```python
from build123d import *

# Parameters (mm, degrees)
SKETCH1_R                   = 60
SKETCH1_R_2                 = 37
BOSS_EXTRUDE1_DEPTH         = 4
F_3_16_0_1875_DOWEL_HOLE1_D = 4.7625


with BuildPart() as part:
    # Sketch1 → Boss-Extrude1 (new body)
    with BuildSketch(Plane.XY):
        Circle(SKETCH1_R)
        Circle(SKETCH1_R_2, mode=Mode.SUBTRACT)
    extrude(amount=BOSS_EXTRUDE1_DEPTH)

    # 3/16 (0.1875) Dowel Hole1 (through all)
    with Locations(Plane(origin=(-54, 0, 4), x_dir=(1, 0, 0), z_dir=(0, 0, 1))):
        with Locations((0, 0), (108, 0), (27, 46.765371804), (27, -46.765371804), (81, 46.765371804), (81, -46.765371804)):
            Hole(F_3_16_0_1875_DOWEL_HOLE1_D / 2)


solid = part.part
```
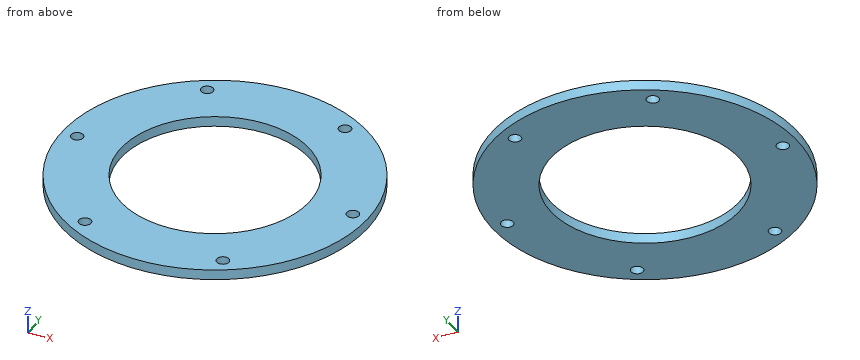
Here's how the part is built. I have some questions about the finished solid (model axes, mm). Coordinates: 2 decimals unless noted, no trailing zeros. Write each loop counter-clockwise with the first axis right and the second up, starting at its lowest first coordinate (ties: lowest second). Pieces come first, ordered by that corner, then holes. Notation, with made-up numbers: (71, 56) - (107, 56) arc R21 ccw to (107, 61) - close; hole circle Ø4 at (18, 36). An arc over 180 degrees is marked (long way). One line per item, written item: value.
1) Suppose I cut it at C-C on y = 0. Write out the boundary of the cut face in (x, z).
Model answer:
outline: (-60, 0) - (-56.38, 0) - (-56.38, 4) - (-60, 4) - close; (-51.62, 0) - (-37, 0) - (-37, 4) - (-51.62, 4) - close; (37, 0) - (51.62, 0) - (51.62, 4) - (37, 4) - close; (56.38, 0) - (60, 0) - (60, 4) - (56.38, 4) - close
2) Suppose I cut it at B-B on y = 16. Write out the boundary of the cut face in (x, z).
Model answer:
outline: (-57.83, 0) - (-33.36, 0) - (-33.36, 4) - (-57.83, 4) - close; (33.36, 0) - (57.83, 0) - (57.83, 4) - (33.36, 4) - close
3) Suppose I cut it at A-A on x = 0. Write out the boundary of the cut face in (y, z).
Model answer:
outline: (-60, 0) - (-37, 0) - (-37, 4) - (-60, 4) - close; (37, 0) - (60, 0) - (60, 4) - (37, 4) - close
4) I need wall thicknesses on line 1 along Y through (x, z) = (1.5, 3); line 2 along Y through (x, z) = (-27, 2.3); line 3 along Y through (x, z) = (-10.5, 2.35). Which ranges of each line are inside material? Lowest first, please.
Model answer:
line 1: y = -59.98 to -36.97, 36.97 to 59.98
line 2: y = -53.58 to -49.15, -44.38 to -25.3, 25.3 to 44.38, 49.15 to 53.58
line 3: y = -59.07 to -35.48, 35.48 to 59.07
5) Suppose I cut it at D-D on x = -27. Write out the boundary of the cut face in (y, z).
Model answer:
outline: (-53.58, 0) - (-49.15, 0) - (-49.15, 4) - (-53.58, 4) - close; (-44.38, 0) - (-25.3, 0) - (-25.3, 4) - (-44.38, 4) - close; (25.3, 0) - (44.38, 0) - (44.38, 4) - (25.3, 4) - close; (49.15, 0) - (53.58, 0) - (53.58, 4) - (49.15, 4) - close
6) I'm going to push flat-ended pins straight in: P1, Ø3, axis at x = 27, y = -46.77, coming from the +Z side; P2, Ø2, axis at y = 21, z = 1, coming from the +X side. Where does each tip first touch, or does it pass through?
Model answer:
P1: passes through
P2: stops at x = 56.57
